Check sheet for the modelled part. Datum: model origin and axes. Units: mm. Face numbers are marked on the shaded views. Give positions to 0.01 mm unless a question says otherwise; leave off trailing zeros. Order: outer loops, then holes, each group sorted by start corner. A loop starts at its lowest first (then second) coordinate and runs counter-clockwise, first axis right, second up.
Item 1: Sectioned sample at B-B on z = 0.8. Record the boundary of the cut face in (x, y).
Item 2: Sectioned sample at A-A on y = 55.5. Record the boundary of the cut face in (x, z), and give its area (3 significant figures).
Item 3: Material ranges on line 1 along X through (y, z) = (54.5, 1.7); line 2 along X through (y, z) = (55, 2.65); line 3 along Y through (x, z) = (81, 2.3) (3 decimals), recorded low to high.
Item 4: Release check for a two-part mould opening along Y. For the marked faces 1, 2, 3 and 4 record: released by +Y, released by -Y, zero draft, split by the parting line, or undercut.
Item 5: Sectioned sample at D-D on x = 83.5. Record the boundary of the cut face in (y, z).
Item 6: Sectioned sample at C-C on y = 51.25. Record the boundary of the cut face in (x, z).
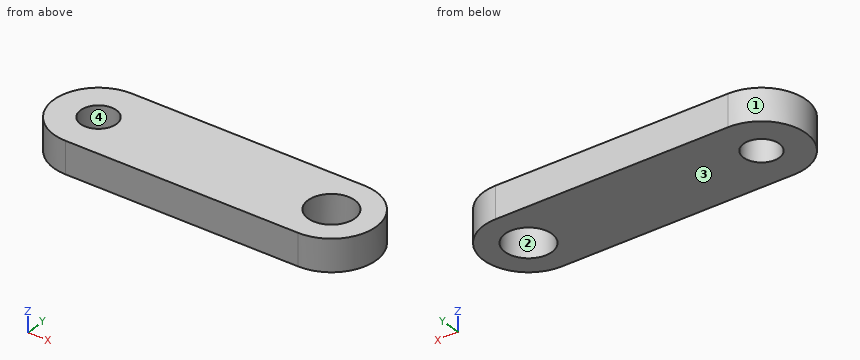
from build123d import *

# Parameters (mm, degrees)
MODEL_R             = 2.199999997
MODEL_R_2           = 1.682352939
BOSS_EXTRUDE1_DEPTH = 3


with BuildPart() as part:
    # Model → Boss-Extrude1 (new body)
    with BuildSketch(Plane.XY):
        with BuildLine():
            Line((64.051409634, 50.149226664), (78.999546271, 50.149226664))
            Line((78.999546271, 50.149226664), (80.881972122, 50.149226664))
            ThreePointArc((80.881972122, 50.149226664), (85.085686549, 54.352941092), (80.881972122, 58.55665552))
            Line((80.881972122, 58.55665552), (58.88197211, 58.55665552))
            ThreePointArc((58.88197211, 58.55665552), (54.678257705, 54.352941069), (58.881972156, 50.149226664))
            Line((58.881972156, 50.149226664), (64.051409634, 50.149226664))
        make_face()
        with Locations((80.881972122, 54.352233082)):
            Circle(MODEL_R, mode=Mode.SUBTRACT)
        with Locations((58.881972133, 54.352941092)):
            Circle(MODEL_R_2, mode=Mode.SUBTRACT)
    extrude(amount=BOSS_EXTRUDE1_DEPTH)


solid = part.part
Report:
1. outline: (58.88, 50.15) - (80.88, 50.15) arc R4.2 ccw to (80.88, 58.56) - (58.88, 58.56) arc R4.2 ccw to start; hole circle Ø3.36 at (58.88, 54.35); hole circle Ø4.4 at (80.88, 54.35)
2. outline: (54.84, 0) - (57.65, 0) - (57.65, 3) - (54.84, 3) - close; (60.11, 0) - (79.01, 0) - (79.01, 3) - (60.11, 3) - close; (82.76, 0) - (84.93, 0) - (84.93, 3) - (82.76, 3) - close
2. area: 71.6 mm2
3. line 1: x = 54.68 to 57.21, 60.56 to 78.69, 83.08 to 85.08
3. line 2: x = 54.73 to 57.33, 60.43 to 78.78, 82.98 to 85.04
3. line 3: y = 50.151 to 52.155, 56.549 to 58.555
4. face 1: split by the parting line
4. face 2: undercut
4. face 3: zero draft
4. face 4: undercut
5. outline: (51.06, 0) - (57.64, 0) - (57.64, 3) - (51.06, 3) - close
6. outline: (56.05, 0) - (83.72, 0) - (83.72, 3) - (56.05, 3) - close
